The model under review builds one solid part; all positions refer to its coordinate system, in mm. A direction names the side the tool comes from. Round coordinates to 2 decimals unless told otherwise and drop trailing zeros. Order: outer loops, then holes, each group sorted by start corner. A loop starts at its lowest first (then second) coordinate and runs counter-clockwise, first axis right, second up.
1) Consider section D-D (z = 3.25). Give the boundary of the cut face in (x, y), then the cut area to 3 significant figures.
2) Clearance check with flat-ended pins moving along their axes: P1, Ø1.4, axis at x = 0, y = 0, coming from the -Z side; P2, Ø2, axis at x = 0.5, y = -1.5, coming from the +Z side; P3, Ø1.5, axis at y = 1, z = 1, coming from the +X side; P4, Ø2, axis at y = -1.5, z = 4, coming from the -X side. State where each tip first meets the part, or that it passes through.
3) To check wall thickness, follow L1, parallel to Z at x = -1.2, y = 0.95; L2, parallel to Z at x = -0.15, y = 0.7; L3, parallel to Y at x = 0.45, z = 6.5. State the ranges of each line that lie inside material, in increasing order.
4) Consider section C-C (z = 9.75). Give the boundary of the cut face in (x, y), then the cut area to 3 significant figures.
5) Consider section A-A (y = 0). Give the boundary of the cut face in (x, z), then the cut area to 3 significant figures.
6) Machinability: for faces 1 (the face through (-1, 1, 5.9)), 2 (the face through (-0.29, 2.23, 4.89)), 3 (the face through (-1, 0, 3.9)), which of the approach directions +Z, -Z, +X, -X, +Y, -Y give a long, thin tool a straight path to every point of the face, cutting with its end or side? Answer none if there is none.
from build123d import *

# Parameters (mm, degrees)
SKETCH1_R           = 0.4
BOSS_EXTRUDE1_DEPTH = 1.1
SKETCH2_R           = 0.65
BOSS_EXTRUDE2_DEPTH = 2.8
SKETCH3_R           = 2.25
BOSS_EXTRUDE3_DEPTH = 2
SKETCH4_R           = 1.15
BOSS_EXTRUDE4_DEPTH = 3
SKETCH5_R           = 0.4
BOSS_EXTRUDE5_DEPTH = 1.1


with BuildPart() as part:
    # Sketch1 → Boss-Extrude1 (new body)
    with BuildSketch(Plane.XY):
        Circle(SKETCH1_R)
    extrude(amount=BOSS_EXTRUDE1_DEPTH)

    # Sketch2 → Boss-Extrude2 (add)
    with BuildSketch(Plane.XY.offset(1.1)):
        Circle(SKETCH2_R)
    extrude(amount=BOSS_EXTRUDE2_DEPTH)

    # Sketch3 → Boss-Extrude3 (add)
    with BuildSketch(Plane.XY.offset(3.9)):
        Circle(SKETCH3_R)
    extrude(amount=BOSS_EXTRUDE3_DEPTH)

    # Sketch4 → Boss-Extrude4 (add)
    with BuildSketch(Plane.XY.offset(5.9)):
        Circle(SKETCH4_R)
    extrude(amount=BOSS_EXTRUDE4_DEPTH)

    # Sketch5 → Boss-Extrude5 (add)
    with BuildSketch(Plane.XY.offset(8.9)):
        Circle(SKETCH5_R)
    extrude(amount=BOSS_EXTRUDE5_DEPTH)


solid = part.part
Answer below:
1. outline: circle Ø1.3 at (0, 0)
1. area: 1.33 mm2
2. P1: stops at z = 0
2. P2: stops at z = 8.9
2. P3: stops at x = 0.6
2. P4: stops at x = -2.19
3. L1: z = 3.9 to 5.9
3. L2: z = 3.9 to 8.9
3. L3: y = -1.06 to 1.06
4. outline: circle Ø0.8 at (0, 0)
4. area: 0.503 mm2
5. outline: (-2.25, 3.9) - (-0.65, 3.9) - (-0.65, 1.1) - (-0.4, 1.1) - (-0.4, 0) - (0.4, 0) - (0.4, 1.1) - (0.65, 1.1) - (0.65, 3.9) - (2.25, 3.9) - (2.25, 5.9) - (1.15, 5.9) - (1.15, 8.9) - (0.4, 8.9) - (0.4, 10) - (-0.4, 10) - (-0.4, 8.9) - (-1.15, 8.9) - (-1.15, 5.9) - (-2.25, 5.9) - close
5. area: 21.3 mm2
6. face 1: +Z
6. face 2: +Z, -Z
6. face 3: -Z
